Design review of the part built by this model. Coordinates are the model's own, in mm. A direction names the side the tool comes from. Round coordinates to 2 decimals unless told otherwise and drop trailing zeros. Loops run counter-clockwise (first coordinate to the right, second up) from the corner with the lowest first, then second, coordinate; pieces in that order, holes last. Notation, with made-up numbers: M 10.25,7.25 L 58.25,7.25 A33 ccw 58.25,36.25 Z; hole C -1,79 d6. An arc over 180 degrees is marked long. One line per item, written item: value. Start each with the question number.
Item 1: For line 1 along Z through (x, y) = (29.5, -2.5); line 2 along Y through (x, z) = (29, 47); line 3 along X through (y, z) = (4.5, 60.5), list the stretches that pass through material, from the lowest coordinate up.
Item 2: For faces 4 (the flat face through (0, 19, 58)), 5 (the flat face through (-2, 39, 58)), list the 3-axis set-ups (+Z, -Z, +X, -X, +Y, -Y) from which the entire face can be reached by the end or side of a thin tool; tool diameter is ignored.
Item 3: Mouldability with a two-part tool opening along Y and no side actions: class faces 1 (the flat face through (-1, 9, 0)), 2 (the flat face through (17, 0, 58)), 3 (the cylindrical face through (-1.97, 37.69, 47.36)) as released by +Y, released by -Y, zero draft, split by the parting line, or undercut.
Item 4: We need section C-C (y = 5). Write out the cut boundary in (x, z).
Item 5: We need section B-B (z = 17). Write out the cut boundary in (x, y), then the cut area to 3 significant figures.
Item 6: Clearance check with flat-ended pins moving along their axes: pin 1 (1.8 mm diameter, centred on x = -2.5, y = -2.5, fed in from -Z); pin 2 (3 mm diameter, centred on y = 36.5, z = 70.8, fed in from +X); pin 3 (2 mm diameter, centred on y = 36.5, z = 47.2, fed in from -X); pin 4 (1.4 mm diameter, centred on x = -2.5, y = 36.5, fed in from -Z). State where each tip first meets the part, or that it passes through.
Item 7: We need section A-A (x = 31). Write out the cut boundary in (y, z).
from build123d import *

# Parameters (mm, degrees)
BOSS_EXTRUDE_EQUERRE_DEPTH                     = 118
FRAISAGE_POUR_VIS_T_TE_FRAIS_E_M20_D           = 2.4
FRAISAGE_POUR_VIS_T_TE_FRAIS_E_M20_DEPTH       = 5
FRAISAGE_POUR_VIS_T_TE_FRAIS_E_M20_CSINK_D     = 4.4
FRAISAGE_POUR_VIS_T_TE_FRAIS_E_M20_CSINK_ANGLE = 90
FRAISAGE_POUR_VIS_T_TE_FRAIS_E_M20_TIP         = 0.721032743
TROU_TARAUD_M2X0_43_D                          = 1.6
TROU_TARAUD_M2X0_43_DEPTH                      = 8
TROU_TARAUD_M2X0_43_TIP                        = 0.480688495
TROU_TARAUD_M2X0_44_AT_2_COUNT                 = 2
TROU_TARAUD_M2X0_44_AT_2_PITCH                 = 39


with BuildPart() as part:
    # Esquisse1 → Boss_Extrude_Equerre (new body)
    with BuildSketch(Plane(origin=(0, 0, 0), x_dir=(0, 1, 0), z_dir=(0, 0, 1))):
        Polygon((0, 0), (39, 0), (39, 5), (-5, 5), (-5, 0), (-5, -34), (0, -34), align=None)
    extrude(amount=BOSS_EXTRUDE_EQUERRE_DEPTH)

    # Fraisage pour vis à tête fraisée M20
    with Locations(Plane.ZY.offset(5)):
        with Locations((70.8, 36.5), (94.4, 36.5), (47.2, 36.5), (23.6, 36.5)):
            CounterSinkHole(FRAISAGE_POUR_VIS_T_TE_FRAIS_E_M20_D / 2, FRAISAGE_POUR_VIS_T_TE_FRAIS_E_M20_CSINK_D / 2, depth=FRAISAGE_POUR_VIS_T_TE_FRAIS_E_M20_DEPTH, counter_sink_angle=FRAISAGE_POUR_VIS_T_TE_FRAIS_E_M20_CSINK_ANGLE)
            with Locations((0, 0, -(FRAISAGE_POUR_VIS_T_TE_FRAIS_E_M20_DEPTH + FRAISAGE_POUR_VIS_T_TE_FRAIS_E_M20_TIP / 2))):  # 118° drill point
                Cone(0, FRAISAGE_POUR_VIS_T_TE_FRAIS_E_M20_D / 2, FRAISAGE_POUR_VIS_T_TE_FRAIS_E_M20_TIP, mode=Mode.SUBTRACT)

    # Trou taraudé M2x0.43
    with Locations(Plane.YZ.offset(34)):
        with Locations((-2.5, 70.8), (-2.5, 94.4), (-2.5, 47.2), (-2.5, 23.6)):
            Hole(TROU_TARAUD_M2X0_43_D / 2, depth=TROU_TARAUD_M2X0_43_DEPTH)
            with Locations((0, 0, -(TROU_TARAUD_M2X0_43_DEPTH + TROU_TARAUD_M2X0_43_TIP / 2))):  # 118° drill point
                Cone(0, TROU_TARAUD_M2X0_43_D / 2, TROU_TARAUD_M2X0_43_TIP, mode=Mode.SUBTRACT)

    # Esquisse11 → Trou taraudé M2x0.44 (revolve, cut)
    with BuildSketch(Plane(origin=(-2.5, 36.5, 118), x_dir=(0, -1, 0), z_dir=(1, 0, 0))):
        Polygon((0, 0), (0, 8.480688495), (0.8, 8), (0.8, 0), align=None)
    trou_taraud_m2x0_44 = revolve(axis=Axis((-2.5, 36.5, 124.35), (0, 0, -1)), mode=Mode.SUBTRACT)

    # Trou taraudé M2x0.44 at 2: Trou taraudé M2x0.44 ×2
    with Locations(*[(0, -i * TROU_TARAUD_M2X0_44_AT_2_PITCH, 0) for i in range(1, TROU_TARAUD_M2X0_44_AT_2_COUNT)]):
        add(trou_taraud_m2x0_44, mode=Mode.SUBTRACT)

    # Symétrie1: Trou taraudé M2x0.44 across plane
    add(trou_taraud_m2x0_44.mirror(Plane.XY.offset(59)), mode=Mode.SUBTRACT)

    # Symétrie1 copy 1 sketch → Symétrie1 copy 1 (revolve, cut)
    with BuildSketch(Plane(origin=(-2.5, -2.5, 0), x_dir=(0, -1, 0), z_dir=(1, 0, 0))):
        Polygon((0, 0), (0, -8.480688495), (0.8, -8), (0.8, 0), align=None)
    revolve(axis=Axis((-2.5, -2.5, -6.35), (0, 0, -1)), mode=Mode.SUBTRACT)


solid = part.part
A:
1. line 1: 0 to 22.8, 24.4 to 46.4, 48 to 70, 71.6 to 93.6, 95.2 to 118
1. line 2: -5 to -3.27, -1.73 to 0
1. line 3: -5 to 0
2. face 4: +Z, -Z, +X, +Y
2. face 5: +Z, -Z, +X, -X, +Y
3. face 1: zero draft
3. face 2: released by +Y
3. face 3: undercut
4. outline: M -5,0 L 0,0 L 0,118 L -5,118 Z
5. outline: M -5,-5 L 34,-5 L 34,0 L 0,0 L 0,39 L -5,39 Z
5. area: 390 mm2
6. pin 1: z = 0
6. pin 2: x = 0
6. pin 3: through
6. pin 4: z = 8.06
7. outline: M -5,0 L 0,0 L 0,118 L -5,118 Z; hole C -2.5,23.6 d1.6; hole C -2.5,47.2 d1.6; hole C -2.5,70.8 d1.6; hole C -2.5,94.4 d1.6
